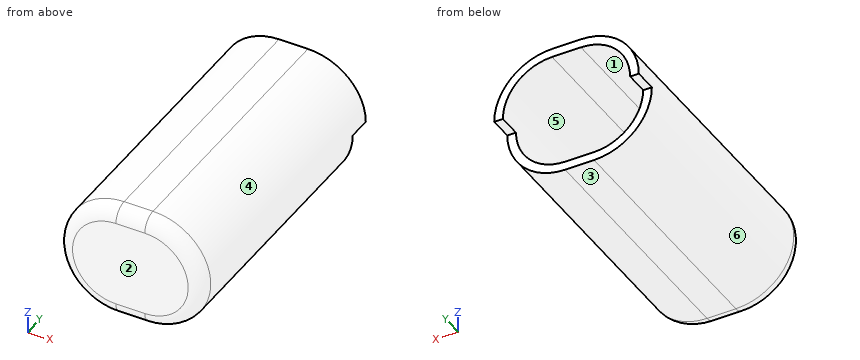
from build123d import *

# Parameters (mm, degrees)
PAD008_DEPTH            = 100
POCKET014_DEPTH         = 97
SKETCH025_W             = 50
SKETCH025_H             = 20
POCKET015_DEPTH         = 8
FILLET001_R             = 5
FILLET002_R             = 5
BODY007_PLACEMENT_ANGLE = 180


with BuildPart() as part:
    # Sketch023 → Pad008 (new body)
    with BuildSketch(Plane.XZ):
        with BuildLine():
            ThreePointArc((-5, 20), (-25, 0), (-5, -20))
            Line((-5, -20), (5, -20))
            ThreePointArc((5, -20), (25, 0), (5, 20))
            Line((5, 20), (-5, 20))
        make_face()
    extrude(amount=PAD008_DEPTH)

    # Sketch024 (on Face6 of Pad008) → Pocket014 (cut)
    with BuildSketch(Plane.XZ.offset(100)):
        with BuildLine():
            ThreePointArc((-5, 17), (-22, 0), (-5, -17))
            Line((-5, -17), (5, -17))
            ThreePointArc((5, -17), (22, 0), (5, 17))
            Line((5, 17), (-5, 17))
        make_face()
    extrude(amount=-POCKET014_DEPTH, mode=Mode.SUBTRACT)

    # Sketch025 (on Face5 of Pocket014) → Pocket015 (cut)
    with BuildSketch(Plane.XZ.offset(100)):
        with Locations((0, -10)):
            Rectangle(SKETCH025_W, SKETCH025_H)
    extrude(amount=-POCKET015_DEPTH, mode=Mode.SUBTRACT)

    # Fillet001
    fillet001_edges = [part.edges().sort_by_distance(p)[0] for p in [
        (-25, 0, 0),
        (0, 0, -20),
        (25, 0, 0),
        (0, 0, 20),
    ]]
    fillet(fillet001_edges, radius=FILLET001_R)

    # Fillet002
    fillet002_edges = [part.edges().sort_by_distance(p)[0] for p in [
        (-22, -3, 0),
        (0, -3, -17),
        (22, -3, 0),
        (0, -3, 17),
    ]]
    fillet(fillet002_edges, radius=FILLET002_R)


with BuildPart() as part_1:
    # Body007 placement: moved
    add(part.part.moved(Location((60, -92.5, 76.5))).rotate(Axis((60, -92.5, 76.5), (0, 0, 1)), BODY007_PLACEMENT_ANGLE))


solid = part_1.part
Part model, mm, in its own coordinate system. Face numbers are marked on the shaded views. A direction names the side the tool comes from. Coordinates: 2 decimals unless noted, no trailing zeros. Order: outer loops, then holes, each group sorted by start corner. A loop starts at its lowest first (then second) coordinate and runs counter-clockwise, first axis right, second up. Notation, with made-up numbers: (-28.75, 74.5) - (9.25, 74.5) arc R17 cw to (9.25, 104.5) - close; hole circle Ø4 at (34.5, 44). An arc over 180 degrees is marked (long way). Use CSV: the item, a comma, the result in double quotes.
Item 1: Mould opens along X. For the marked faces 3, 4, 5 and 6 say: +X half, -X half, draft (parallel to the pull), parting line (faces both ways), or undercut.
Solved:
face 3,"draft"
face 4,"+X half"
face 5,"undercut"
face 6,"-X half"
Item 2: Probe probe 1 along X at (y, z) = (-36, 76.5); probe 2 along Y at (x, z) = (67.5, 73); probe 3 along Z at (x, y) = (77, -12). List the from-to ranges inside material, lowest first.
Solved:
probe 1,"x = 35 to 38, 82 to 85"
probe 2,"y = -92.5 to -89.5"
probe 3,"z = 60.5 to 64.46, 88.54 to 92.5"
Item 3: Drop flat-ended pins along their axis: P1, Ø0.9, axis at x = 83, y = 1.5, coming from the -Z side; P2, Ø3, axis at x = 75, z = 60.5, coming from the -Y side; P3, Ø10, axis at x = 60.5, z = 62, coming from the +Y side. Give the stop position or say it passes through.
Solved:
P1,"stops at z = 76.5"
P2,"stops at y = -91.9"
P3,"stops at y = -0.5"
Item 4: Saw through at A-A on y = -36.5. Give the cut face in (x, z), and give its area (3 significant figures).
Solved:
outline,"(55, 56.5) - (65, 56.5) arc R20 ccw to (65, 96.5) - (55, 96.5) arc R20 ccw to start; hole (55, 59.5) - (65, 59.5) arc R17 ccw to (65, 93.5) - (55, 93.5) arc R17 ccw to start"
area,"409 mm²"
Item 5: 3-axis set-ups, long thin cutter, end or side, ignore diameter. For the marked faces 1 and 2: which of +Z, -Z, +X, -X, +Y, -Y reach the whole face in a straight line?
Solved:
face 1,"+Y"
face 2,"+Z, -Z, +X, -X, -Y"
